```python
from build123d import *

# Parameters (mm, degrees)
SKETCH1_W             = 1750
SKETCH1_H             = 1750
SKETCH1_W_2           = 1670
SKETCH1_H_2           = 525
SKETCH1_H_3           = 775
BOSS_EXTRUDE1_DEPTH   = 40
SKETCH2_W             = 40
SKETCH2_H             = 40
BOSS_EXTRUDE2_DEPTH   = 1160
SKETCH3_W             = 40
SKETCH3_H             = 40
BOSS_EXTRUDE3_DEPTH   = 1710
SKETCH4_W             = 40
SKETCH4_H             = 40
BOSS_EXTRUDE4_DEPTH   = 1710
SKETCH5_W             = 40
SKETCH5_H             = 40
BOSS_EXTRUDE5_DEPTH   = 1710
SKETCH6_W             = 950
SKETCH6_H             = 40
CUT_EXTRUDE1_DEPTH    = 40
SKETCH9_W             = 290
SKETCH9_H             = 40
CUT_EXTRUDE4_DEPTH    = 40
M8_TAPPED_HOLE1_D     = 6.8
M8_TAPPED_HOLE1_DEPTH = 17.707073895
M8_TAPPED_HOLE1_TIP   = 2.042926105
SKETCH13_W            = 40
SKETCH13_H            = 40
BOSS_EXTRUDE6_DEPTH   = 1710
SKETCH15_W            = 815
SKETCH15_H            = 40
CUT_EXTRUDE5_DEPTH    = 40
SKETCH16_W            = 40
SKETCH16_H            = 40
BOSS_EXTRUDE7_DEPTH   = 815
SKETCH18_R            = 3.3
CUT_EXTRUDE6_DEPTH    = 40
SKETCH20_R            = 3.3
CUT_EXTRUDE8_DEPTH    = 40
SKETCH22_W            = 40
SKETCH22_H            = 40
BOSS_EXTRUDE8_DEPTH   = 330
SKETCH23_R            = 4.5
CUT_EXTRUDE9_DEPTH    = 40


with BuildPart() as part:
    # Sketch1 → Boss-Extrude1 (new body)
    with BuildSketch(Plane(origin=(0, 0, 0), x_dir=(1, 0, 0), z_dir=(0, 1, 0))):
        Rectangle(SKETCH1_W, SKETCH1_H)
        with Locations((0, 572.5)):
            Rectangle(SKETCH1_W_2, SKETCH1_H_2, mode=Mode.SUBTRACT)
        with Locations((0, -447.5)):
            Rectangle(SKETCH1_W_2, SKETCH1_H_3, mode=Mode.SUBTRACT)
        Polygon((-835, -20), (835, -20), (835, 20), (835, 270), (-835, 270), (-835, 20), align=None, mode=Mode.SUBTRACT)
    extrude(amount=BOSS_EXTRUDE1_DEPTH)

    # Sketch2 → Boss-Extrude2 (add)
    with BuildSketch(Plane.XZ):
        with Locations((-855, 855)):
            Rectangle(SKETCH2_W, SKETCH2_H)
        with Locations((855, 855)):
            Rectangle(SKETCH2_W, SKETCH2_H)
        with Locations((0, 855)):
            Rectangle(SKETCH2_W, SKETCH2_H)
        with Locations((855, 40)):
            Rectangle(SKETCH2_W, SKETCH2_H)
        with Locations((-855, 40)):
            Rectangle(SKETCH2_W, SKETCH2_H)
        with Locations((-855, -855)):
            Rectangle(SKETCH2_W, SKETCH2_H)
        with Locations((855, -855)):
            Rectangle(SKETCH2_W, SKETCH2_H)
        with Locations((495, -855)):
            Rectangle(SKETCH2_W, SKETCH2_H)
        with Locations((-495, -855)):
            Rectangle(SKETCH2_W, SKETCH2_H)
        with Locations((-855, -290)):
            Rectangle(SKETCH2_W, SKETCH2_H)
        with Locations((855, -290)):
            Rectangle(SKETCH2_W, SKETCH2_H)
    extrude(amount=BOSS_EXTRUDE2_DEPTH)

    # Sketch3 → Boss-Extrude3 (add)
    with BuildSketch(Plane.XY.offset(875)):
        with Locations((-855, -535)):
            Rectangle(SKETCH3_W, SKETCH3_H)
        with Locations((855, -535)):
            Rectangle(SKETCH3_W, SKETCH3_H)
    extrude(amount=-BOSS_EXTRUDE3_DEPTH)

    # Sketch4 → Boss-Extrude4 (add)
    with BuildSketch(Plane.ZY.offset(875)):
        with Locations((855, -535)):
            Rectangle(SKETCH4_W, SKETCH4_H)
    extrude(amount=-BOSS_EXTRUDE4_DEPTH)

    # Sketch5 → Boss-Extrude5 (add)
    with BuildSketch(Plane.ZY.offset(875)):
        with Locations((-855, -535)):
            Rectangle(SKETCH5_W, SKETCH5_H)
    extrude(amount=-BOSS_EXTRUDE5_DEPTH)

    # Sketch6 → Cut-Extrude1 (cut)
    with BuildSketch(Plane(origin=(0, 0, -875), x_dir=(-1, 0, 0), z_dir=(0, 0, -1))):
        with Locations((0, -535)):
            Rectangle(SKETCH6_W, SKETCH6_H)
    extrude(amount=-CUT_EXTRUDE1_DEPTH, mode=Mode.SUBTRACT)

    # Sketch9 → Cut-Extrude4 (cut)
    with BuildSketch(Plane.ZY.offset(875)):
        with Locations((-125, -535)):
            Rectangle(SKETCH9_W, SKETCH9_H)
    extrude(amount=-CUT_EXTRUDE4_DEPTH, mode=Mode.SUBTRACT)

    # M8 Tapped Hole1
    with Locations(Plane(origin=(0, 40, 0), x_dir=(1, 0, 0), z_dir=(0, 1, 0))):
        with Locations((85, -40), (-85, -40), (-85, 290), (85, 290)):
            Hole(M8_TAPPED_HOLE1_D / 2, depth=M8_TAPPED_HOLE1_DEPTH)
            with Locations((0, 0, -(M8_TAPPED_HOLE1_DEPTH + M8_TAPPED_HOLE1_TIP / 2))):  # 118° drill point
                Cone(0, M8_TAPPED_HOLE1_D / 2, M8_TAPPED_HOLE1_TIP, mode=Mode.SUBTRACT)

    # Sketch13 → Boss-Extrude6 (add)
    with BuildSketch(Plane(origin=(875, 0, 0), x_dir=(0, 0, -1), z_dir=(1, 0, 0))):
        with Locations((-40, -415)):
            Rectangle(SKETCH13_W, SKETCH13_H)
        with Locations((290, -415)):
            Rectangle(SKETCH13_W, SKETCH13_H)
        with Locations((-855, -415)):
            Rectangle(SKETCH13_W, SKETCH13_H)
    extrude(amount=-BOSS_EXTRUDE6_DEPTH)

    # Sketch15 → Cut-Extrude5 (cut)
    with BuildSketch(Plane.XY.offset(875)):
        with Locations((-427.5, -415)):
            Rectangle(SKETCH15_W, SKETCH15_H)
    extrude(amount=-CUT_EXTRUDE5_DEPTH, mode=Mode.SUBTRACT)

    # Sketch16 → Boss-Extrude7 (add)
    with BuildSketch(Plane.XY.offset(875)):
        with Locations((400, -415)):
            Rectangle(SKETCH16_W, SKETCH16_H)
    extrude(amount=-BOSS_EXTRUDE7_DEPTH)

    # Sketch18 → Cut-Extrude6 (cut)
    with BuildSketch(Plane(origin=(0, -395, 0), x_dir=(1, 0, 0), z_dir=(0, 1, 0))):
        with Locations((400, -275)):
            Circle(SKETCH18_R)
    extrude(amount=-CUT_EXTRUDE6_DEPTH, mode=Mode.SUBTRACT)

    # Sketch20 → Cut-Extrude8 (cut)
    with BuildSketch(Plane(origin=(0, -395, 0), x_dir=(1, 0, 0), z_dir=(0, 1, 0))):
        with Locations((651.445575403, -40)):
            Circle(SKETCH20_R)
        with Locations((651.445575403, 290)):
            Circle(SKETCH20_R)
    extrude(amount=-CUT_EXTRUDE8_DEPTH, mode=Mode.SUBTRACT)

    # Sketch22 → Boss-Extrude8 (add)
    with BuildSketch(Plane.XY.offset(60)):
        with Locations((495, -415)):
            Rectangle(SKETCH22_W, SKETCH22_H)
        with Locations((310.857864376, -415)):
            Rectangle(SKETCH22_W, SKETCH22_H)
    extrude(amount=-BOSS_EXTRUDE8_DEPTH)

    # Sketch23 → Cut-Extrude9 (cut)
    with BuildSketch(Plane(origin=(0, -395, 0), x_dir=(1, 0, 0), z_dir=(0, 1, 0))):
        with Locations((310.857864376, 125)):
            Circle(SKETCH23_R)
        with Locations((495, 125)):
            Circle(SKETCH23_R)
    extrude(amount=-CUT_EXTRUDE9_DEPTH, mode=Mode.SUBTRACT)


solid = part.part
```
Work out the finished part from the listing and answer in its coordinate system (mm). A direction names the side the tool comes from. Give positions to 0.01 mm unless a question says otherwise; leave off trailing zeros. Order: outer loops, then holes, each group sorted by start corner. A loop starts at its lowest first (then second) coordinate and runs counter-clockwise, first axis right, second up. Notation, with made-up numbers: (-7, 81) - (17, 81) arc R20 cw to (17, 119) - close; hole circle Ø3 at (48.5, 40). An arc over 180 degrees is marked (long way). One line per item, written item: value. Start each with the question number.
1. Section A-A, the plane x = -220 is taken. Write down the section's boundary in (y, z), then the cut area to 3 significant figures.
2. For a pull along Z with two mould halves and no side action, classify faces 1 (the face through (-875, 21, -4)), 2 (the face through (835, -635, 58)), 3 (the face through (514, -429, -875)) as released by +Z, released by -Z, zero draft, split by the parting line, or undercut.
3. Each of these flat-tipped pins is pushed along its axis until it touches: pin 1 Ø20 at (y, z) = (-415.5, 456.5) entering from +X; pin 2 Ø4 at (x, z) = (400, 275) entering from +Y; pin 3 Ø8 at (x, z) = (-85, 40) entering from -Y. Where does it stop, or does it pass through?
4. Section D-D, the plane z = -645.5 is taken. Write down the section's boundary in (x, y).
5. Section B-B, the plane z = 752 is taken. Write down the section's boundary in (x, y).
6. Section C-C, the plane x = -580 is taken. Count the separate pieces of the cut face and the enclosed holes in it, then the cut area to 3 significant figures.
7. Consider line 1 (Z direction, x = 85, y = 27.5); line 2 (X direction, y = 32.75, z = -290); line 3 (Z direction, x = 400, y = -416). Determine where each line is inside the solid, lowest interval first.
8. Which of the six approach directions +Z, -Z, +X, -X, +Y, -Y give full straight-line access (tool end or side, diameter ignored) to faces 4 (the face through (-554, -405, 20)), 5 (the face through (748, -409, 60)), 6 (the face through (-835, -554, -428))?
Filled sheet:
1. outline: (-555, 835) - (-515, 835) - (-515, 875) - (-555, 875) - close; (-435, -310) - (-395, -310) - (-395, -270) - (-435, -270) - close; (-435, 20) - (-395, 20) - (-395, 60) - (-435, 60) - close; (0, -875) - (40, -875) - (40, -835) - (0, -835) - close; (0, -310) - (40, -310) - (40, -270) - (0, -270) - close; (0, 20) - (40, 20) - (40, 60) - (0, 60) - close; (0, 835) - (40, 835) - (40, 875) - (0, 875) - close
1. area: 11,200 mm²
2. face 1: zero draft
2. face 2: undercut
2. face 3: released by -Z
3. pin 1: x = 420
3. pin 2: through
3. pin 3: y = -435
4. outline: (-875, -555) - (-835, -555) - (-835, -515) - (-875, -515) - close; (-875, 0) - (-835, 0) - (-835, 40) - (-875, 40) - close; (835, -555) - (875, -555) - (875, -515) - (835, -515) - close; (835, 0) - (875, 0) - (875, 40) - (835, 40) - close
5. outline: (-875, -555) - (-835, -555) - (-835, -515) - (-875, -515) - close; (-875, 0) - (-835, 0) - (-835, 40) - (-875, 40) - close; (380, -435) - (420, -435) - (420, -395) - (380, -395) - close; (835, -555) - (875, -555) - (875, -515) - (835, -515) - close; (835, 0) - (875, 0) - (875, 40) - (835, 40) - close
6. separate pieces: 8
6. enclosed holes: 0
6. area: 12,800 mm²
7. line 1: -875 to -835, -310 to -293.4, -286.6 to -270, 20 to 36.6, 43.4 to 60, 835 to 875
7. line 2: -875 to -88.4, -81.6 to 81.6, 88.4 to 875
7. line 3: -310 to -270, 20 to 271.7, 278.3 to 875
8. face 4: -X, -Y
8. face 5: +X
8. face 6: -Y
